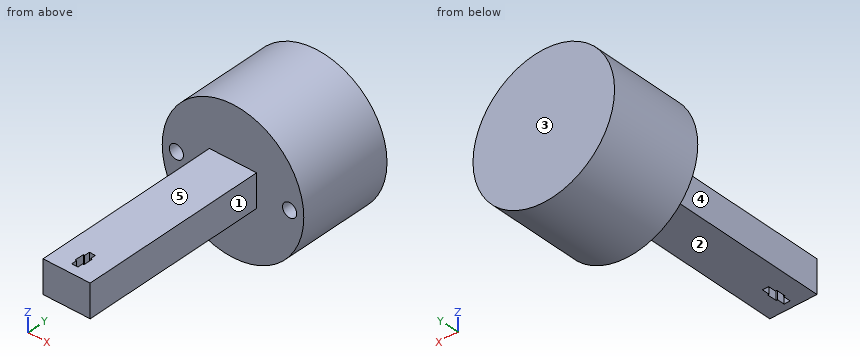
```python
from build123d import *

# Parameters (mm, degrees)
SKETCH_1_R          = 15
EXTRUDE_1_DEPTH     = 20
SKETCH_2_R          = 1.5
CUT_EXTRUDE_1_DEPTH = 15
SKETCH_3_W          = 10
SKETCH_3_H          = 7
EXTRUDE_2_DEPTH     = 40
SKETCH_4_W          = 1.3
SKETCH_4_H          = 4.2
CUT_EXTRUDE_2_DEPTH = 47.75467891
SKETCH_5_W          = 1.3
SKETCH_5_H          = 5.2
CUT_EXTRUDE_3_DEPTH = 2
SKETCH_6_W          = 1.9
SKETCH_6_H          = 2
CUT_EXTRUDE_4_DEPTH = 47.75467891


with BuildPart() as part:
    # 草图1 → 凸台-拉伸1 (new body)
    with BuildSketch(Plane(origin=(0, 0, 0), x_dir=(1, 0, 0), z_dir=(0, 1, 0))):
        with Locations(Location((0, 0, 0), (0, 0, 270))):
            Circle(SKETCH_1_R)
    extrude(amount=EXTRUDE_1_DEPTH)

    # 草图2 → 切除-拉伸1 (cut)
    with BuildSketch(Plane.XZ):
        with Locations(Location((12, 0, 0), (0, 0, 270))):
            Circle(SKETCH_2_R)
        with Locations(Location((-12, 0, 0), (0, 0, 90))):
            Circle(SKETCH_2_R)
    extrude(amount=-CUT_EXTRUDE_1_DEPTH, mode=Mode.SUBTRACT)

    # 草图3 → 凸台-拉伸2 (add)
    with BuildSketch(Plane.XZ):
        with Locations((0, 0.5)):
            Rectangle(SKETCH_3_W, SKETCH_3_H)
    extrude(amount=EXTRUDE_2_DEPTH)

    # 草图4 → 切除-拉伸2 (cut, through all)
    with BuildSketch(Plane.XY.offset(4)):
        with Locations((0, -35.9)):
            Rectangle(SKETCH_4_W, SKETCH_4_H)
    extrude(amount=-CUT_EXTRUDE_2_DEPTH, mode=Mode.SUBTRACT)

    # 草图5 → 切除-拉伸3 (cut)
    with BuildSketch(Plane.XY.offset(-3)):
        with Locations((0, -35.9)):
            Rectangle(SKETCH_5_W, SKETCH_5_H)
    extrude(amount=CUT_EXTRUDE_3_DEPTH, mode=Mode.SUBTRACT)

    # 草图6 → 切除-拉伸4 (cut, through all)
    with BuildSketch(Plane.XY.offset(4)):
        with Locations((0, -35.9)):
            Rectangle(SKETCH_6_W, SKETCH_6_H)
    extrude(amount=-CUT_EXTRUDE_4_DEPTH, mode=Mode.SUBTRACT)


solid = part.part
```
Work out the finished part from the listing and answer in its coordinate system (mm). Face numbers are marked on the shaded views. A direction names the side the tool comes from. Coordinates: 2 decimals unless noted, no trailing zeros. Write each loop counter-clockwise with the first axis right and the second up, starting at its lowest first coordinate (ties: lowest second). Pieces come first, ordered by that corner, then holes.
Q1. Each of these flat-tipped pins is pushed along its axis until it touches: pin 1 Ø3.5 at (y, z) = (-16, 1) entering from +X; pin 2 Ø6 at (x, y) = (-9.5, -30.5) entering from +Z (3 decimals); pin 3 Ø1 at (y, z) = (0, -6.5) entering from -X; pin 4 Ø1 at (y, z) = (8, -3) entering from -X. Where does it stop, or does it pass through?
Q2. A cutting plane is placed at D-D, the plane x = 12. Give the vertices of the cut face in (y, z).
Q3. A cutting plane is placed at C-C, the plane z = 0. Give the vertices of the cut face in (x, y).
Q4. Which of the six approach directions +Z, -Z, +X, -X, +Y, -Y give full straight-line access (tool end or side, diameter ignored) to the marked faces 1, 2, 3, 4 and 5?
Q5. Find the intervals of material crossed by line 1 (X direction, y = 12.25, z = 0); line 2 (Y direction, x = 0.25, z = -1.25); line 3 (Y direction, x = 4.25, z = -5.75), in increasing order.
Q6. A cutting plane is placed at A-A, the plane x = 0. Give the vertices of the cut face in (y, z), then the cut area to 3 significant figures.
Q7. A cutting plane is placed at B-B, the plane y = -35.5. Give the vertices of the cut face in (x, z).
Findings below:
1. pin 1: stops at x = 5
1. pin 2: passes through
1. pin 3: stops at x = -13.75
1. pin 4: stops at x = -14.79
2. outline: (0, -9) - (20, -9) - (20, 9) - (0, 9) - (0, 1.5) - (15, 1.5) - (15, -1.5) - (0, -1.5) - close
3. outline: (-15, 0) - (-13.5, 0) - (-13.5, 15) - (-10.5, 15) - (-10.5, 0) - (-5, 0) - (-5, -40) - (5, -40) - (5, 0) - (10.5, 0) - (10.5, 15) - (13.5, 15) - (13.5, 0) - (15, 0) - (15, 20) - (-15, 20) - close; hole (-0.95, -36.9) - (-0.65, -36.9) - (-0.65, -38) - (0.65, -38) - (0.65, -36.9) - (0.95, -36.9) - (0.95, -34.9) - (0.65, -34.9) - (0.65, -33.8) - (-0.65, -33.8) - (-0.65, -34.9) - (-0.95, -34.9) - close
4. face 1: +Z, -Z, +X, -Y
4. face 2: -Z, +X, -X, -Y
4. face 3: +Z, -Z, +X, -X, +Y
4. face 4: +Z, -Z, -X, -Y
4. face 5: +Z, +X, -X, -Y
5. line 1: x = -15 to -13.5, -10.5 to 10.5, 13.5 to 15
5. line 2: y = -40 to -38.5, -33.3 to 20
5. line 3: y = 0 to 20
6. outline: (-40, -3) - (-38.5, -3) - (-38.5, -1) - (-38, -1) - (-38, 4) - (-40, 4) - close; (-33.8, -1) - (-33.3, -1) - (-33.3, -3) - (0, -3) - (0, -15) - (20, -15) - (20, 15) - (0, 15) - (0, 4) - (-33.8, 4) - close
6. area: 849 mm2
7. outline: (-5, -3) - (-0.95, -3) - (-0.95, 4) - (-5, 4) - close; (0.95, -3) - (5, -3) - (5, 4) - (0.95, 4) - close
